Here's how the part is built. I have some questions about the finished solid (model axes, mm). A direction names the side the tool comes from. Round coordinates to 2 decimals unless told otherwise and drop trailing zeros. Order: outer loops, then holes, each group sorted by start corner. A loop starts at its lowest first (then second) coordinate and runs counter-clockwise, first axis right, second up. Notation, with made-up numbers: (22, -13.5) - (28, -13.5) arc R19 cw to (28, 13.5) - close; hole circle Ø11 at (2.5, -3). An arc over 180 degrees is marked (long way). Answer as a JSON object with one key per item and string values.
```python
from build123d import *

# Parameters (mm, degrees)
BOSS_EXTRUDE1_DEPTH = 9.5
SKETCH2_R           = 1.5
CUT_EXTRUDE1_DEPTH  = 19
SKETCH3_R           = 1.5
CUT_EXTRUDE2_DEPTH  = 19
FILLET1_R           = 5


with BuildPart() as part:
    # Sketch1 → Boss-Extrude1 (new, symmetric)
    with BuildSketch(Plane.XY):
        Polygon((0, 0), (0, 9), (2, 9), (2, 2), (10, 2), (10, 0), align=None)
    extrude(amount=BOSS_EXTRUDE1_DEPTH, both=True)

    # Sketch2 → Cut-Extrude1 (cut)
    with BuildSketch(Plane(origin=(0, 2, 0), x_dir=(1, 0, 0), z_dir=(0, 1, 0))):
        with Locations(Location((6.5, 5, 0), (0, 0, 270))):
            Circle(SKETCH2_R)
        with Locations(Location((6.5, -5, 0), (0, 0, 270))):
            Circle(SKETCH2_R)
    extrude(amount=-CUT_EXTRUDE1_DEPTH, mode=Mode.SUBTRACT)

    # Sketch3 → Cut-Extrude2 (cut)
    with BuildSketch(Plane(origin=(2, 0, 0), x_dir=(0, 0, -1), z_dir=(1, 0, 0))):
        with Locations(Location((0, 5.5, 0), (0, 0, 90))):
            Circle(SKETCH3_R)
    extrude(amount=-CUT_EXTRUDE2_DEPTH, mode=Mode.SUBTRACT)

    # Fillet1
    fillet1_edges = [part.edges().sort_by_distance(p)[0] for p in [
        (1, 9, 9.5),
        (1, 9, -9.5),
    ]]
    fillet(fillet1_edges, radius=FILLET1_R)


solid = part.part
```
1. Thinking about a two-plate mould opening in Y: for faces 1 (the face through (1, 4, 0)), 2 (the face through (1.01, 7.5, -8.07)), 3 (the face through (5.17, 1.01, 5.69)), which applies, pulls with the +Y half, pulls with the -Y half, needs draft (parallel to the pull), parting line crosses it, or undercut?
Responses:
{"face 1": "undercut", "face 2": "pulls with the +Y half", "face 3": "needs draft"}
2. For faces 4 (the face through (6, 2, 0)), 5 (the face through (1.01, 7.5, 8.07)), which set-ups out of +Z, -Z, +X, -X, +Y, -Y let a thin tool reach every point of the face, with its end or its side?
Responses:
{"face 4": "+Z, -Z, +X, +Y", "face 5": "+Z, +X, -X, +Y"}
3. For P1, Ø4, axis at y = 2, z = -0.5, coming from the -X side; P2, Ø1.5, axis at x = 7.5, z = -2, coming from the +Y side, each with a flat end and sliding along its axis, tell me the tip position at first contact or that it passes through.
Responses:
{"P1": "x = 0", "P2": "y = 2"}
4. Imagine slicing it at C-C (y = 5). List the corners of the cut face in (x, z) for me.
Responses:
{"outline": "(0, -9.4) - (2, -9.4) - (2, -1.41) - (0, -1.41) - close; (0, 1.41) - (2, 1.41) - (2, 9.4) - (0, 9.4) - close"}
5. Imagine slicing it at D-D (y = 1.5). List the corners of the cut face in (x, z) for me, plus the area to 3 significant figures.
Responses:
{"outline": "(0, -9.5) - (10, -9.5) - (10, 9.5) - (0, 9.5) - close; hole circle Ø3 at (6.5, -5); hole circle Ø3 at (6.5, 5)", "area": "176 mm2"}
6. Imagine slicing it at A-A (x = 1.25). List the corners of the cut face in (y, z) for me, plus the area to 3 significant figures.
Responses:
{"outline": "(0, -9.5) - (4, -9.5) arc R5 ccw to (9, -4.5) - (9, 4.5) arc R5 ccw to (4, 9.5) - (0, 9.5) - close; hole circle Ø3 at (5.5, 0)", "area": "153 mm2"}
7. If I drill on L1, parallel to X at y = 1.35, z = -5; L2, parallel to X at y = 6.5, z = 6, over which ranges is the centre line in solid material (lowest first)? Write a range as [from, to].
Responses:
{"L1": "[0, 5], [8, 10]", "L2": "[0, 2]"}
8. Imagine slicing it at B-B (z = 0). List the corners of the cut face in (x, y) for me, plus the area to 3 significant figures.
Responses:
{"outline": "(0, 0) - (10, 0) - (10, 2) - (2, 2) - (2, 4) - (0, 4) - close; (0, 7) - (2, 7) - (2, 9) - (0, 9) - close", "area": "28.0 mm2"}
